Work out the finished part from the listing and answer in its coordinate system (mm). A direction names the side the tool comes from. Coordinates: 2 decimals unless noted, no trailing zeros. Order: outer loops, then holes, each group sorted by start corner. A loop starts at its lowest first (then second) coordinate and runs counter-clockwise, first axis right, second up. Notation, with made-up numbers: M 51,3.5 L 72,3.5 A26 ccw 72,38.5 Z; hole C -40,-32.5 d6. An arc over 180 degrees is marked long. Answer in a Markdown table with one row per item. Add a question column.
Item 1: Flat-ended cylindrical pins translate along their axes: pin 1 Ø9 at (x, y) = (-13, 3.5) entering from +Z; pin 2 Ø1 at (x, z) = (4.5, 5) entering from +Y; pin 3 Ø4.5 at (y, z) = (-5, 6.5) entering from +X. Find the tip coordinate at first contact, or state that the pin passes through.
Item 2: The part is cut by section A-A (y = 0). Write down the section's boundary in (x, z).
Item 3: Consider line 1 (Z direction, x = 0, y = 4); line 2 (Z direction, x = 6.5, y = -9.5); line 3 (X direction, y = -14, z = 6). Determine where each line is inside the solid, lowest interval first. Write a range as from..to.
Item 4: The mould has two halves that part along X. Classify faces 1 (the face through (0, 0, 3)), 2 (the face through (-3.47, -15.62, 3.99)), 3 (the face through (4, 0, 0)): released by +X, released by -X, zero draft, split by the parting line, or undercut.
Item 5: The part is cut by section D-D (y = -14). Write down the section's boundary in (x, z).
Item 6: Which of the six approach directions +Z, -Z, +X, -X, +Y, -Y give full straight-line access (tool end or side, diameter ignored) to faces 4 (the face through (1, 0, 1)), 5 (the face through (7.7, -14.2, 3)), 6 (the face through (9, 0, 5)), 7 (the face through (-9, 0, 5))?
Item 7: The part is cut by section B-B (x = 0). Write down the section's boundary in (y, z).
Item 8: The part is cut by section C-C (z = 4.5). Write down the section's boundary in (x, y), then the cut area to 3 significant figures.
from build123d import *

# Parameters (mm, degrees)
F0_R     = 17.5
F1_DEPTH = 3
F2_R     = 16
F3_DEPTH = 2
F5_DEPTH = 4
F6_W     = 2
F6_H     = 10
F7_DEPTH = 3


with BuildPart() as f1:
    # F0 (on Top) → F1 (new body)
    with BuildSketch(Plane.XY):
        Circle(F0_R)
    extrude(amount=F1_DEPTH)

    # F2 (on face) → F3 (join)
    with BuildSketch(Plane.XY.offset(3)):
        Circle(F2_R)
    extrude(amount=F3_DEPTH)

    # F4 (on face) → F5 (join)
    with BuildSketch(Plane.XY.offset(5)):
        with BuildLine():
            Line((4.5, -16.911535), (4.5, 16.911535))
            ThreePointArc((4.5, 16.911535), (0, 17.5), (-4.5, 16.911535))
            Line((-4.5, 16.911535), (-4.5, -16.911535))
            ThreePointArc((-4.5, -16.911535), (0, -17.5), (4.5, -16.911535))
        make_face()
    extrude(amount=F5_DEPTH)

    # F6 (on face) → F7 (cut)
    with BuildSketch(Plane(origin=(0, 0, 0), x_dir=(1, 0, 0), z_dir=(0, 0, -1))):
        Rectangle(F6_W, F6_H)
    extrude(amount=-F7_DEPTH, mode=Mode.SUBTRACT)


solid = f1.part
Reply:
| question | item | result |
|---|---|---|
| 1 | pin 1 | stops at z = 5 |
| 1 | pin 2 | stops at y = 17.04 |
| 1 | pin 3 | stops at x = 15.65 |
| 2 | outline | M -17.5,0 L -1,0 L -1,3 L 1,3 L 1,0 L 17.5,0 L 17.5,3 L 16,3 L 16,5 L 4.5,5 L 4.5,9 L -4.5,9 L -4.5,5 L -16,5 L -16,3 L -17.5,3 Z |
| 3 | line 1 | z = 3..9 |
| 3 | line 2 | z = 0..5 |
| 3 | line 3 | x = -4.5..4.5 |
| 4 | face 1 | undercut |
| 4 | face 2 | split by the parting line |
| 4 | face 3 | zero draft |
| 5 | outline | M -10.5,0 L 10.5,0 L 10.5,3 L 7.75,3 L 7.75,5 L 4.5,5 L 4.5,9 L -4.5,9 L -4.5,5 L -7.75,5 L -7.75,3 L -10.5,3 Z |
| 6 | face 4 | -Z |
| 6 | face 5 | none |
| 6 | face 6 | +Z, +X, +Y, -Y |
| 6 | face 7 | +Z, -X, +Y, -Y |
| 7 | outline | M -17.5,0 L -5,0 L -5,3 L 5,3 L 5,0 L 17.5,0 L 17.5,3 L 16,3 L 16,5 L 17.5,5 L 17.5,9 L -17.5,9 L -17.5,5 L -16,5 L -16,3 L -17.5,3 Z |
| 8 | outline | C 0,0 d32 |
| 8 | area | 804 mm2 |
